from build123d import *

# Parameters (mm, degrees)
SKETCH1_W           = 60
SKETCH1_H           = 50
BOSS_EXTRUDE1_DEPTH = 2.5
SKETCH2_W           = 8
SKETCH2_H           = 2
BOSS_EXTRUDE2_DEPTH = 10
CUT_EXTRUDE1_REACH  = 44.252
SKETCH3_R           = 3.05
SKETCH4_W           = 8
SKETCH4_H           = 2
BOSS_EXTRUDE3_DEPTH = 10
CUT_EXTRUDE2_REACH  = 44.252
SKETCH6_R           = 3.05
SKETCH7_W           = 8
SKETCH7_H           = 4
BOSS_EXTRUDE4_DEPTH = 10
CUT_EXTRUDE3_REACH  = 44.252
SKETCH8_R           = 3.05
SKETCH9_W           = 8
SKETCH9_H           = 2
BOSS_EXTRUDE5_DEPTH = 10
CUT_EXTRUDE4_REACH  = 56.261
SKETCH10_R          = 3.05
CUT_EXTRUDE5_REACH  = 56.261
SKETCH12_R          = 3.05
CUT_EXTRUDE6_REACH  = 56.261
SKETCH13_R          = 3.05
CUT_EXTRUDE7_REACH  = 56.261
SKETCH14_R          = 3.05
CUT_EXTRUDE8_REACH  = 42.311
SKETCH15_W          = 8
SKETCH15_H          = 5.36479905


with BuildPart() as part:
    # Sketch1 → Boss-Extrude1 (new body)
    with BuildSketch(Plane(origin=(0, 0, 0), x_dir=(1, 0, 0), z_dir=(0, 1, 0))):
        Rectangle(SKETCH1_W, SKETCH1_H)
    extrude(amount=BOSS_EXTRUDE1_DEPTH)

    # Sketch2 → Boss-Extrude2 (add)
    with BuildSketch(Plane(origin=(0, 2.5, 0), x_dir=(1, 0, 0), z_dir=(0, 1, 0))):
        with Locations((-25, -1)):
            Rectangle(SKETCH2_W, SKETCH2_H)
    extrude(amount=BOSS_EXTRUDE2_DEPTH)

    # Sketch3 → Cut-Extrude1 (cut, up to next)
    with BuildSketch(Plane.XY.offset(2), mode=Mode.PRIVATE) as cut_extrude1_sk1:
        with Locations((-25, 7.5)):
            Circle(SKETCH3_R)
    cut_extrude1_tool1 = extrude(cut_extrude1_sk1.sketch, amount=-CUT_EXTRUDE1_REACH, mode=Mode.PRIVATE) & part.part
    add(cut_extrude1_tool1.solids().sort_by_distance((-25, 7.5, 2))[0], mode=Mode.SUBTRACT)

    # Sketch4 → Boss-Extrude3 (add)
    with BuildSketch(Plane(origin=(0, 2.5, 0), x_dir=(1, 0, 0), z_dir=(0, 1, 0))):
        with Locations((-25, 1)):
            Rectangle(SKETCH4_W, SKETCH4_H)
    extrude(amount=BOSS_EXTRUDE3_DEPTH)

    # Sketch6 → Cut-Extrude2 (cut, up to next)
    with BuildSketch(Plane(origin=(0, 0, -2), x_dir=(-1, 0, 0), z_dir=(0, 0, -1)), mode=Mode.PRIVATE) as cut_extrude2_sk1:
        with Locations(Location((25, 7.5, 0), (0, 0, 180))):
            Circle(SKETCH6_R)
    cut_extrude2_tool1 = extrude(cut_extrude2_sk1.sketch, amount=-CUT_EXTRUDE2_REACH, mode=Mode.PRIVATE) & part.part
    add(cut_extrude2_tool1.solids().sort_by_distance((-25, 7.5, -2))[0], mode=Mode.SUBTRACT)

    # Sketch7 → Boss-Extrude4 (add)
    with BuildSketch(Plane(origin=(0, 2.5, 0), x_dir=(1, 0, 0), z_dir=(0, 1, 0))):
        with Locations((25, 0)):
            Rectangle(SKETCH7_W, SKETCH7_H)
    extrude(amount=BOSS_EXTRUDE4_DEPTH)

    # Sketch8 → Cut-Extrude3 (cut, up to next)
    with BuildSketch(Plane.XY.offset(2), mode=Mode.PRIVATE) as cut_extrude3_sk1:
        with Locations((25, 7.5)):
            Circle(SKETCH8_R)
    cut_extrude3_tool1 = extrude(cut_extrude3_sk1.sketch, amount=-CUT_EXTRUDE3_REACH, mode=Mode.PRIVATE) & part.part
    add(cut_extrude3_tool1.solids().sort_by_distance((25, 7.5, 2))[0], mode=Mode.SUBTRACT)

    # Sketch9 → Boss-Extrude5 (add)
    with BuildSketch(Plane(origin=(0, 2.5, 0), x_dir=(1, 0, 0), z_dir=(0, 1, 0))):
        with Locations((-25, 17.450740252)):
            Rectangle(SKETCH9_W, SKETCH9_H)
        with Locations((-25, -17.450740252)):
            Rectangle(SKETCH9_W, SKETCH9_H)
        with Locations((25, -17.450740252)):
            Rectangle(SKETCH9_W, SKETCH9_H)
        with Locations((25, 17.450740252)):
            Rectangle(SKETCH9_W, SKETCH9_H)
    extrude(amount=BOSS_EXTRUDE5_DEPTH)

    # Sketch10 → Cut-Extrude4 (cut, up to next)
    with BuildSketch(Plane(origin=(0, 0, -18.450740252), x_dir=(-1, 0, 0), z_dir=(0, 0, -1)), mode=Mode.PRIVATE) as cut_extrude4_sk1:
        with Locations(Location((25, 7.5, 0), (0, 0, 180))):
            Circle(SKETCH10_R)
    cut_extrude4_tool1 = extrude(cut_extrude4_sk1.sketch, amount=-CUT_EXTRUDE4_REACH, mode=Mode.PRIVATE) & part.part
    add(cut_extrude4_tool1.solids().sort_by_distance((-25, 7.5, -18.45074))[0], mode=Mode.SUBTRACT)

    # Sketch12 → Cut-Extrude5 (cut, up to next)
    with BuildSketch(Plane.XY.offset(18.450740252), mode=Mode.PRIVATE) as cut_extrude5_sk1:
        with Locations((-25, 7.5)):
            Circle(SKETCH12_R)
    cut_extrude5_tool1 = extrude(cut_extrude5_sk1.sketch, amount=-CUT_EXTRUDE5_REACH, mode=Mode.PRIVATE) & part.part
    add(cut_extrude5_tool1.solids().sort_by_distance((-25, 7.5, 18.45074))[0], mode=Mode.SUBTRACT)

    # Sketch13 → Cut-Extrude6 (cut, up to next)
    with BuildSketch(Plane(origin=(0, 0, -18.450740252), x_dir=(-1, 0, 0), z_dir=(0, 0, -1)), mode=Mode.PRIVATE) as cut_extrude6_sk1:
        with Locations(Location((-25, 7.5, 0), (0, 0, 180))):
            Circle(SKETCH13_R)
    cut_extrude6_tool1 = extrude(cut_extrude6_sk1.sketch, amount=-CUT_EXTRUDE6_REACH, mode=Mode.PRIVATE) & part.part
    add(cut_extrude6_tool1.solids().sort_by_distance((25, 7.5, -18.45074))[0], mode=Mode.SUBTRACT)

    # Sketch14 → Cut-Extrude7 (cut, up to next)
    with BuildSketch(Plane.XY.offset(18.450740252), mode=Mode.PRIVATE) as cut_extrude7_sk1:
        with Locations((25, 7.5)):
            Circle(SKETCH14_R)
    cut_extrude7_tool1 = extrude(cut_extrude7_sk1.sketch, amount=-CUT_EXTRUDE7_REACH, mode=Mode.PRIVATE) & part.part
    add(cut_extrude7_tool1.solids().sort_by_distance((25, 7.5, 18.45074))[0], mode=Mode.SUBTRACT)

    # Sketch15 → Cut-Extrude8 (cut, up to next)
    with BuildSketch(Plane(origin=(0, 2.5, 0), x_dir=(1, 0, 0), z_dir=(0, 1, 0)), mode=Mode.PRIVATE) as cut_extrude8_sk1:
        with Locations((-25, 21.133139777)):
            Rectangle(SKETCH15_W, SKETCH15_H)
    cut_extrude8_tool1 = extrude(cut_extrude8_sk1.sketch, amount=-CUT_EXTRUDE8_REACH, mode=Mode.PRIVATE) & part.part
    # Sketch15 → Cut-Extrude8 (cut, up to next)
    with BuildSketch(Plane(origin=(0, 2.5, 0), x_dir=(1, 0, 0), z_dir=(0, 1, 0)), mode=Mode.PRIVATE) as cut_extrude8_sk2:
        with Locations((25, 21.133139777)):
            Rectangle(SKETCH15_W, SKETCH15_H)
    cut_extrude8_tool2 = extrude(cut_extrude8_sk2.sketch, amount=-CUT_EXTRUDE8_REACH, mode=Mode.PRIVATE) & part.part
    # Sketch15 → Cut-Extrude8 (cut, up to next)
    with BuildSketch(Plane(origin=(0, 2.5, 0), x_dir=(1, 0, 0), z_dir=(0, 1, 0)), mode=Mode.PRIVATE) as cut_extrude8_sk3:
        with Locations((-25, -21.133139777)):
            Rectangle(SKETCH15_W, SKETCH15_H)
    cut_extrude8_tool3 = extrude(cut_extrude8_sk3.sketch, amount=-CUT_EXTRUDE8_REACH, mode=Mode.PRIVATE) & part.part
    # Sketch15 → Cut-Extrude8 (cut, up to next)
    with BuildSketch(Plane(origin=(0, 2.5, 0), x_dir=(1, 0, 0), z_dir=(0, 1, 0)), mode=Mode.PRIVATE) as cut_extrude8_sk4:
        with Locations((25, -21.133139777)):
            Rectangle(SKETCH15_W, SKETCH15_H)
    cut_extrude8_tool4 = extrude(cut_extrude8_sk4.sketch, amount=-CUT_EXTRUDE8_REACH, mode=Mode.PRIVATE) & part.part
    add(cut_extrude8_tool1.solids().sort_by_distance((-25, 2.5, -21.13314))[0], mode=Mode.SUBTRACT)
    add(cut_extrude8_tool2.solids().sort_by_distance((25, 2.5, -21.13314))[0], mode=Mode.SUBTRACT)
    add(cut_extrude8_tool3.solids().sort_by_distance((-25, 2.5, 21.13314))[0], mode=Mode.SUBTRACT)
    add(cut_extrude8_tool4.solids().sort_by_distance((25, 2.5, 21.13314))[0], mode=Mode.SUBTRACT)


solid = part.part
Verification items for the finished model (mm, model axes). A direction names the side the tool comes from. Give positions to 0.01 mm unless a question says otherwise; leave off trailing zeros. Write each loop counter-clockwise with the first axis right and the second up, starting at its lowest first coordinate (ties: lowest second). Pieces come first, ordered by that corner, then holes. Notation, with made-up numbers: M 55,66.5 L 62,66.5 A28 ccw 62,87.5 Z; hole C -29,2.25 d4. An arc over 180 degrees is marked long. Use CSV: the item, a comma, the result in double quotes.
1) Cross-section at A-A (z = 19.5). Enter the section's corners in (x, y).
Final values:
outline,"M -30,0 L -29,0 L -29,2.5 L -30,2.5 Z; M -21,0 L 21,0 L 21,2.5 L -21,2.5 Z; M 29,0 L 30,0 L 30,2.5 L 29,2.5 Z"
2) Cross-section at B-B (x = -25). State how many separate pieces and enclosed holes the cut face has, plus the area to 3 significant figures.
Final values:
separate pieces,"6"
enclosed holes,"0"
area,"129 mm²"
3) Cross-section at D-D (z = 12). Enter the section's corners in (x, y).
Final values:
outline,"M -30,0 L 30,0 L 30,2.5 L -30,2.5 Z"
4) Access from +Z, -Z, +X, -X, +Y, -Y to the whole of each face (thin tool, end or side, straight path). Record for faces 4 (the face through (25, 4, -2)), 5 (the face through (-29, 7, -17)), 6 (the face through (-25, 1, -23.816)), 7 (the face through (29, 7, -17)), 8 (the face through (21, 7, 17)).
Final values:
face 4,"+X, -X, +Y"
face 5,"+Z, -Z, -X, +Y"
face 6,"+Y, -Y"
face 7,"+Z, -Z, +X, +Y"
face 8,"+Z, -Z, +Y"
5) Go/stop test with flat-tipped pins: pin 1 Ø25 at (x, z) = (4.5, -4.5) entering from +Y; pin 2 Ø2.5 at (x, y) = (26, 6.5) entering from +Z; pin 3 Ø4 at (x, y) = (26, 8.5) entering from -Z; pin 4 Ø4.5 at (y, z) = (7.5, 0) entering from -X. Record where each tip stops, or that it passes through.
Final values:
pin 1,"y = 2.5"
pin 2,"through"
pin 3,"z = -18.45"
pin 4,"x = -29"
6) Material ranges on line 1 along X through (y, z) = (7.5, -16.95); line 2 along Y through (x, z) = (25, 17.9); line 3 along Y through (x, z) = (-17, 22), recorded low to high.
Final values:
line 1,"-29 to -28.05, -21.95 to -21, 21 to 21.95, 28.05 to 29"
line 2,"0 to 4.45, 10.55 to 12.5"
line 3,"0 to 2.5"
7) Release check for a two-part mould opening along Y. For faces 1 (the face through (25, 12.5, -17)), 2 (the face through (-25, 4, 2)), 3 (the face through (-22.183, 8.668, -0.028)) record: released by +Y, released by -Y, zero draft, split by the parting line, or undercut.
Final values:
face 1,"released by +Y"
face 2,"zero draft"
face 3,"undercut"
